```python
from build123d import *

# Parameters (mm, degrees)
F1_DEPTH      = 381
F1_DEPTH_BACK = 381


with BuildPart() as f1:
    # F0 (on Top) → F1 (new body, two sides)
    with BuildSketch(Plane.XY) as f1_sk:
        with BuildLine():
            ThreePointArc((12.7, 9.525), (11.770064, 11.770064), (9.525, 12.7))
            Line((9.525, 12.7), (-9.525, 12.7))
            ThreePointArc((-9.525, 12.7), (-11.770064, 11.770064), (-12.7, 9.525))
            Line((-12.7, 9.525), (-12.7, -9.525))
            ThreePointArc((-12.7, -9.525), (-11.770064, -11.770064), (-9.525, -12.7))
            Line((-9.525, -12.7), (9.525, -12.7))
            ThreePointArc((9.525, -12.7), (11.770064, -11.770064), (12.7, -9.525))
            Line((12.7, -9.525), (12.7, 9.525))
        make_face()
        with BuildLine():
            Line((-9.525, -6.35), (-9.525, 6.35))
            ThreePointArc((-9.525, 6.35), (-8.595064, 8.595064), (-6.35, 9.525))
            Line((-6.35, 9.525), (6.35, 9.525))
            ThreePointArc((6.35, 9.525), (8.595064, 8.595064), (9.525, 6.35))
            Line((9.525, 6.35), (9.525, -6.35))
            ThreePointArc((9.525, -6.35), (8.595064, -8.595064), (6.35, -9.525))
            Line((6.35, -9.525), (-6.35, -9.525))
            ThreePointArc((-6.35, -9.525), (-8.595064, -8.595064), (-9.525, -6.35))
        make_face(mode=Mode.SUBTRACT)
    extrude(amount=F1_DEPTH)
    extrude(f1_sk.sketch, amount=-F1_DEPTH_BACK)


solid = f1.part
```
Work out the finished part from the listing and answer in its coordinate system (mm). A direction names the side the tool comes from. Coordinates: 2 decimals unless noted, no trailing zeros. Loops run counter-clockwise (first coordinate to the right, second up) from the corner with the lowest first, then second, coordinate; pieces in that order, holes last.
1) For faces 1 (the flat face through (0, 12.7, 5)), 2 (the flat face through (0, 9.525, 5)), determine the directions among +Z, -Z, +X, -X, +Y, -Y from which every point of the face is accessible in a straight line to the end or side of a thin tool.
Results:
face 1: +Z, -Z, +X, -X, +Y
face 2: +Z, -Z
2) A flat-ended cylindrical pin translates along its axis: pin 1 (8 mm diameter, centred on x = 2.5, y = 4.5, fed in from +Z) (3 decimals). Find the tip coordinate at first contact, or state that the pin passes through.
Results:
pin 1: passes through
3) Section C-C (z = -96) is taken. Give the vertices of the cut face in (x, y) (3 decimals), plus the area to 3 significant figures.
Results:
outline: (-12.7, -9.525) arc R3.175 ccw to (-9.525, -12.7) - (9.525, -12.7) arc R3.175 ccw to (12.7, -9.525) - (12.7, 9.525) arc R3.175 ccw to (9.525, 12.7) - (-9.525, 12.7) arc R3.175 ccw to (-12.7, 9.525) - close; hole (-9.525, -6.35) arc R3.175 ccw to (-6.35, -9.525) - (6.35, -9.525) arc R3.175 ccw to (9.525, -6.35) - (9.525, 6.35) arc R3.175 ccw to (6.35, 9.525) - (-6.35, 9.525) arc R3.175 ccw to (-9.525, 6.35) - close
area: 282 mm2
4) Section A-A (x = 2) is taken. Give the vertices of the cut face in (y, z) (3 decimals).
Results:
outline: (-12.7, -381) - (-9.525, -381) - (-9.525, 381) - (-12.7, 381) - close; (9.525, -381) - (12.7, -381) - (12.7, 381) - (9.525, 381) - close
5) Consider probe 1 along X at (y, z) = (0.75, 11) (3 decimals); probe 2 along Y at (x, z) = (8.75, -118.5). Determine where each line is inside the solid, lowest interval first.
Results:
probe 1: x = -12.7 to -9.525, 9.525 to 12.7
probe 2: y = -12.7 to -8.43, 8.43 to 12.7
6) For a pull along Y with two mould halves and no side action, classify faces 3 (the flat face through (-12.7, 0, 5)), 4 (the flat face through (-9.525, 0, 5)), 5 (the flat face through (9.525, 0, 5)), 6 (the flat face through (0, -12.7, 5)) as +Y half, -Y half, draft (parallel to the pull), parting line (faces both ways), or undercut.
Results:
face 3: draft
face 4: undercut
face 5: undercut
face 6: -Y half
